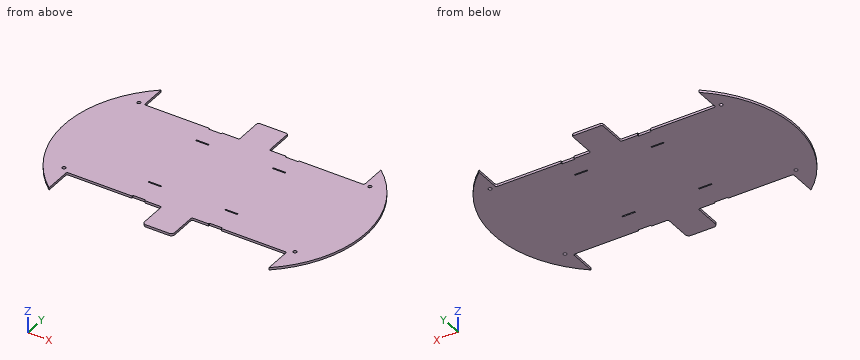
from build123d import *

# Parameters (mm, degrees)
SZKIC1_R                    = 1.5
SZKIC1_W                    = 11
SZKIC1_H                    = 1.1
DODANIE_WYCI_GNI_CIE3_DEPTH = 2


with BuildPart() as part:
    # Szkic1 → Dodanie-wyciągnięcie3 (new body)
    with BuildSketch(Plane.XY):
        with BuildLine():
            Line((-139.727293062, -79.5), (-120.189002398, -79.5))
            ThreePointArc((-120.189002398, -79.5), (-117.912369122, -78.544329486), (-117, -76.25))
            Line((-117, -76.25), (-117, -54.98069498))
            ThreePointArc((-117, -54.98069498), (-116.639537786, -54.110462214), (-115.76930502, -53.75))
            Line((-115.76930502, -53.75), (-102.427025017, -53.75))
            Line((-102.427025017, -53.75), (-102.427025017, -52.65))
            Line((-102.427025017, -52.65), (-91.427025017, -52.65))
            Line((-91.427025017, -52.65), (-91.427025017, -53.75))
            Line((-91.427025017, -53.75), (-87.218924948, -53.75))
            Line((-87.218924948, -53.75), (-36.25, -53.75))
            ThreePointArc((-36.25, -53.75), (-35.366116524, -54.116116524), (-35, -55))
            Line((-35, -55), (-35, -77.5))
            ThreePointArc((-35, -77.5), (0, -2.5), (-35, 72.5))
            Line((-35, 72.5), (-35, 51.25))
            ThreePointArc((-35, 51.25), (-35.366116524, 50.366116524), (-36.25, 50))
            Line((-36.25, 50), (-91.427025017, 50))
            Line((-91.427025017, 50), (-91.427025017, 48.9))
            Line((-91.427025017, 48.9), (-102.427025017, 48.9))
            Line((-102.427025017, 48.9), (-102.427025017, 50))
            Line((-102.427025017, 50), (-115.75, 50))
            ThreePointArc((-115.75, 50), (-116.633883476, 50.366116524), (-117, 51.25))
            Line((-117, 51.25), (-117, 73.75))
            ThreePointArc((-117, 73.75), (-117.366116524, 74.633883476), (-118.25, 75))
            Line((-118.25, 75), (-141.75, 75))
            ThreePointArc((-141.75, 75), (-142.633883476, 74.633883476), (-143, 73.75))
            Line((-143, 73.75), (-143, 51.25))
            ThreePointArc((-143, 51.25), (-143.366116524, 50.366116524), (-144.25, 50))
            Line((-144.25, 50), (-157.572974983, 50))
            Line((-157.572974983, 50), (-157.572974983, 48.9))
            Line((-157.572974983, 48.9), (-168.572974983, 48.9))
            Line((-168.572974983, 48.9), (-168.572974983, 50))
            Line((-168.572974983, 50), (-223.75, 50))
            ThreePointArc((-223.75, 50), (-224.633883476, 50.366116524), (-225, 51.25))
            Line((-225, 51.25), (-225, 72.5))
            ThreePointArc((-225, 72.5), (-260, -2.5), (-225, -77.5))
            Line((-225, -77.5), (-225, -55))
            ThreePointArc((-225, -55), (-224.633883476, -54.116116524), (-223.75, -53.75))
            Line((-223.75, -53.75), (-172.781075052, -53.75))
            Line((-172.781075052, -53.75), (-168.572974983, -53.75))
            Line((-168.572974983, -53.75), (-168.572974983, -52.65))
            Line((-168.572974983, -52.65), (-166.090308712, -52.65))
            Line((-166.090308712, -52.65), (-157.572974983, -52.65))
            Line((-157.572974983, -52.65), (-157.572974983, -53.75))
            Line((-157.572974983, -53.75), (-144.25, -53.75))
            ThreePointArc((-144.25, -53.75), (-143.366116524, -54.116116524), (-143, -55))
            Line((-143, -55), (-143, -76.237644119))
            ThreePointArc((-143, -76.237644119), (-142.040816528, -78.548140635), (-139.727293062, -79.5))
        make_face()
        with Locations((-229.818345238, 50.110219647)):
            Circle(SZKIC1_R, mode=Mode.SUBTRACT)
        with Locations((-229.818345238, -49.889780353)):
            Circle(SZKIC1_R, mode=Mode.SUBTRACT)
        with Locations(Location((-30.181654762, -49.889780353, 0), (0, 0, 180))):
            Circle(SZKIC1_R, mode=Mode.SUBTRACT)
        with Locations(Location((-30.181654762, 50.110219647, 0), (0, 0, 180))):
            Circle(SZKIC1_R, mode=Mode.SUBTRACT)
        with Locations((-163.072974983, -31.85)):
            Rectangle(SZKIC1_W, SZKIC1_H, mode=Mode.SUBTRACT)
        with Locations((-163.072974983, 31.85)):
            Rectangle(SZKIC1_W, SZKIC1_H, mode=Mode.SUBTRACT)
        with Locations((-96.927025017, 31.85)):
            Rectangle(SZKIC1_W, SZKIC1_H, mode=Mode.SUBTRACT)
        with Locations((-96.927025017, -31.85)):
            Rectangle(SZKIC1_W, SZKIC1_H, mode=Mode.SUBTRACT)
    extrude(amount=DODANIE_WYCI_GNI_CIE3_DEPTH)


solid = part.part
Read the model definition and answer for the solid it produces. Units are mm, in the model's axes. Round coordinates to 2 decimals unless told otherwise and drop trailing zeros. Loops run counter-clockwise (first coordinate to the right, second up) from the corner with the lowest first, then second, coordinate; pieces in that order, holes last. Notation, with made-up numbers: (59, -18.5) - (71, -18.5) arc R14 cw to (71, -12.5) - close; hole circle Ø8 at (46.25, 27.5). An arc over 180 degrees is marked (long way). One line per question, with ' | ' between items. Start each with the question number.
Q1. Find the intervals of material crossed by L1, parallel to Y at x = -159, z = 1.4; L2, parallel to X at y = -50.5, z = 1.35; L3, parallel to X at y = -32, z = 1.5, in increasing order.
Q2. Section D-D on y = 35.5 is taken. Give the vertices of the cut face in (x, z), plus the area to 3 significant figures.
Q3. Flat-ended cylindrical pins translate along their axes: pin 1 (1 mm diameter, centred on x = -170.5, z = 1.5, fed in from +Y); pin 2 (1.2 mm diameter, centred on y = -53, z = 1, fed in from -X); pin 3 (0.6 mm diameter, centred on y = -53, z = 1, fed in from +X). Find the tip coordinate at first contact, or state that the pin passes through.
Q4. Section B-B on y = -63 is taken. Give the vertices of the cut face in (x, z).
Q5. Section C-C on z = 1 is taken. Count the separate pieces of the cut face and the enclosed holes in it, plus the area to 3 significant figures.
Q6. Section A-A on x = -99 is taken. Give the vertices of the cut face in (y, z), plus the area to 3 significant figures.
Established:
1) L1: -52.65 to -32.4, -31.3 to 31.3, 32.4 to 48.9 | L2: -247.42 to -231.19, -228.45 to -31.55, -28.81 to -12.58 | L3: -255.45 to -168.57, -157.57 to -102.43, -91.43 to -4.55
2) outline: (-252.32, 0) - (-7.68, 0) - (-7.68, 2) - (-252.32, 2) - close | area: 489 mm²
3) pin 1: y = 50 | pin 2: x = -246.32 | pin 3: x = -13.86
4) outline: (-239.06, 0) - (-225, 0) - (-225, 2) - (-239.06, 2) - close; (-143, 0) - (-117, 0) - (-117, 2) - (-143, 2) - close; (-35, 0) - (-20.94, 0) - (-20.94, 2) - (-35, 2) - close
5) separate pieces: 1 | enclosed holes: 8 | area: 28,200 mm²
6) outline: (-52.65, 0) - (-32.4, 0) - (-32.4, 2) - (-52.65, 2) - close; (-31.3, 0) - (31.3, 0) - (31.3, 2) - (-31.3, 2) - close; (32.4, 0) - (48.9, 0) - (48.9, 2) - (32.4, 2) - close | area: 199 mm²
